Autodesk Inventor part; units mm, degrees
ref_plane "YZ Plane" through (0, 0, 0) normal (1, 0, 0) x (0, 1, 0)
ref_plane "XZ Plane" through (0, 0, 0) normal (0, 1, 0) x (-1, 0, 0)
ref_plane "XY Plane" through (0, 0, 0) normal (0, 0, 1) x (1, 0, 0)
sketch "Sketch1" plane through (0, 0, 0) normal (0, 0, 1) x (1, 0, 0)
  line L0 (0, 0) -> (0, 25.4)
  line L1 (0, 25.4) -> (76.2, 25.4)
  line L2 (76.2, 25.4) -> (76.2, 0)
  line L3 (76.2, 0) -> (63.5, -25.4)
  line L4 (63.5, -25.4) -> (38.1, -25.4)
  line L5 (38.1, -25.4) -> (0, 0)
  dimension "d1" = 25.4
  dimension "d2" = 25.4
  dimension "d3" = 25.4
  dimension "d4" = 76.2
  dimension "d5" = 50.8
  dimension "d6" = 38.1
extrude "Extrusion1" add sketch "Sketch1" along normal blind 3.175
sketch "Sketch2" plane through (0, 0, 3.175) normal (0, 0, 1) x (1, 0, 0)
  line L0 (0, 25.4) -> (0, 0)
  line L1 (38.1, -25.4) -> (63.5, -25.4)
  line L2 (76.2, -25.4) -> (76.2, 25.4)
  line L3 (76.2, 25.4) -> (0, 25.4)
  point P0 (76.2, 0)
  point P1 (12.7, 12.7)
  point P2 (63.5, 12.7)
  point P3 (50.8, -12.7)
  dimension "d9" = 12.7
  dimension "d10" = 12.7
  dimension "d11" = 12.7
  dimension "d12" = 12.7
  dimension "d13" = 12.7
  dimension "d14" = 12.7
  dimension "d22" = 52.3634
hole "Hole1" at (12.7, 12.7, 3.175) at (63.5, 12.7, 3.175) at (50.8, -12.7, 3.175) direction (0, 0, -1) diameter 6.35 end through all
properties part number "TriangleBracket" material "Aluminum 6061"
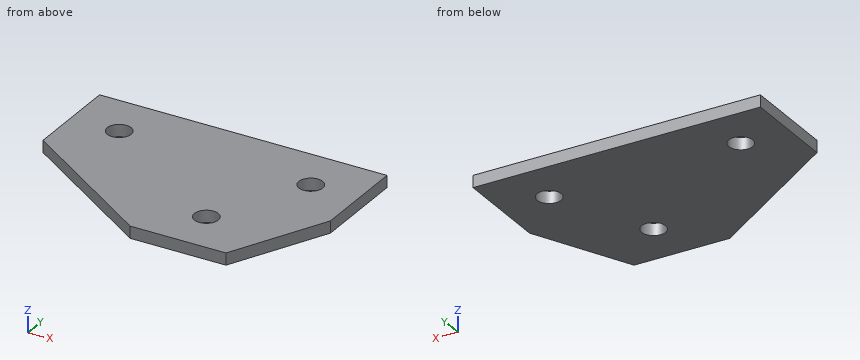
Here's how the part is built. I have some questions about the finished solid (model axes, mm). Give positions to 0.01 mm unless a question says otherwise; leave off trailing zeros. Order: outer loops, then holes, each group sorted by start corner. A loop starts at its lowest first (then second) coordinate and runs counter-clockwise, first axis right, second up. Notation, with made-up numbers: M 8,80 L 40,80 A17 ccw 40,91 Z; hole C -14.75,42.5 d6. An arc over 180 degrees is marked long. Use a Markdown table: item, result. Add a question column.
1. Suppose I cut it at C-C (z = 0.8). List the corners of the cut face in (x, y) for me (3 decimals), and give its area (3 significant figures).
2. For pin 1 Ø1 at (y, z) = (-12, 1.5) entering from +X, with a flat end and sliding along its axis, tell me the tip position at first contact or that it passes through.
3. Suppose I cut it at A-A (y = 12.7). List the corners of the cut face in (x, z) for me (3 decimals).
4. I need wall thicknesses on probe 1 along X at (y, z) = (12.7, 2.05) (3 decimals); probe 2 along Y at (x, z) = (63.5, 1) (3 decimals); probe 3 along X at (y, z) = (15.5, 0.65). Which ranges of each line are inside material? Lowest first, please. Write a range as from..to.
5. Suppose I cut it at B-B (y = -12.7). List the corners of the cut face in (x, z) for me (3 decimals), and give its area (3 significant figures).
6. Suppose I cut it at D-D (x = 12.7). List the corners of the cut face in (y, z) for me (3 decimals).
Results list:
| question | item | result |
|---|---|---|
| 1 | outline | M 0,0 L 38.1,-25.4 L 63.5,-25.4 L 76.2,0 L 76.2,25.4 L 0,25.4 Z; hole C 12.7,12.7 d6.35; hole C 50.8,-12.7 d6.35; hole C 63.5,12.7 d6.35 |
| 1 | area | 3,130 mm² |
| 2 | pin 1 | stops at x = 70.45 |
| 3 | outline | M 0,0 L 9.525,0 L 9.525,3.175 L 0,3.175 Z; M 15.875,0 L 60.325,0 L 60.325,3.175 L 15.875,3.175 Z; M 66.675,0 L 76.2,0 L 76.2,3.175 L 66.675,3.175 Z |
| 4 | probe 1 | x = 0..9.525, 15.875..60.325, 66.675..76.2 |
| 4 | probe 2 | y = -25.4..9.525, 15.875..25.4 |
| 4 | probe 3 | x = 0..11.2, 14.2..62, 65..76.2 |
| 5 | outline | M 19.05,0 L 47.625,0 L 47.625,3.175 L 19.05,3.175 Z; M 53.975,0 L 69.85,0 L 69.85,3.175 L 53.975,3.175 Z |
| 5 | area | 141 mm² |
| 6 | outline | M -8.467,0 L 9.525,0 L 9.525,3.175 L -8.467,3.175 Z; M 15.875,0 L 25.4,0 L 25.4,3.175 L 15.875,3.175 Z |
